Geometry check sheet. Reference: drawing and pictorial views, mm from the part's lowest x, y, z. A direction names the side the tool comes from. Give positions to 0.01 mm unless a question says otherwise; leave off trailing zeros. Write each loop counter-clockwise with the first axis right and the second up, starting at its lowest first coordinate (ties: lowest second). Pieces come first, ordered by that corner, then holes. Notation, with made-up numbers: M -13.5,-7.5 L 37.5,-7.5 A21 ccw 37.5,5.5 Z; hole C 88,55 d10. An arc over 180 degrees is marked long. One line per item, written item: value. Start each with the question number.
1. Cross-section at A-A on x = 14. Record the cut outline in (y, z).
2. Cross-section at B-B on z = 20.5. Record the cut outline in (x, y), then the cut area to 3 significant figures.
3. Scan lines: line 1 (X direction, y = 20.4, z = 10); line 2 (Y direction, x = 4.75, z = 17); line 3 (Z direction, x = 15, y = 26). Record each from-to range of solid material in increasing order.
4. Gauge pin test, flat ends, axial feed: pin 1 (11.5 mm diameter, centred on x = 14, z = 10, fed in from -Y); pin 2 (4.5 mm diameter, centred on y = 22, z = 16, fed in from +X); pin 3 (3 mm diameter, centred on x = 20, y = 17, fed in from -Z); pin 4 (3 mm diameter, centred on x = 13.5, z = 8.5, fed in from -Y). Record the tip position at first contact, or that the pin passes through.
5. Tool access check on the marked faces 4, 5 and 6. Record the directions out of +Z, -Z, +X, -X, +Y, -Y that give a thin tool (end or side, any length) a straight path to the whole face; none if there is none.
6. Cross-section at D-D on y = 21. Record the cut outline in (x, z).
7. Cross-section at C-C on z = 11. Record the cut outline in (x, y).
8. Release check for a two-part mould opening along Y. For the marked faces 1, 2 and 3 record: pulls with the +Y half, pulls with the -Y half, needs draft (parallel to the pull), parting line crosses it, or undercut.
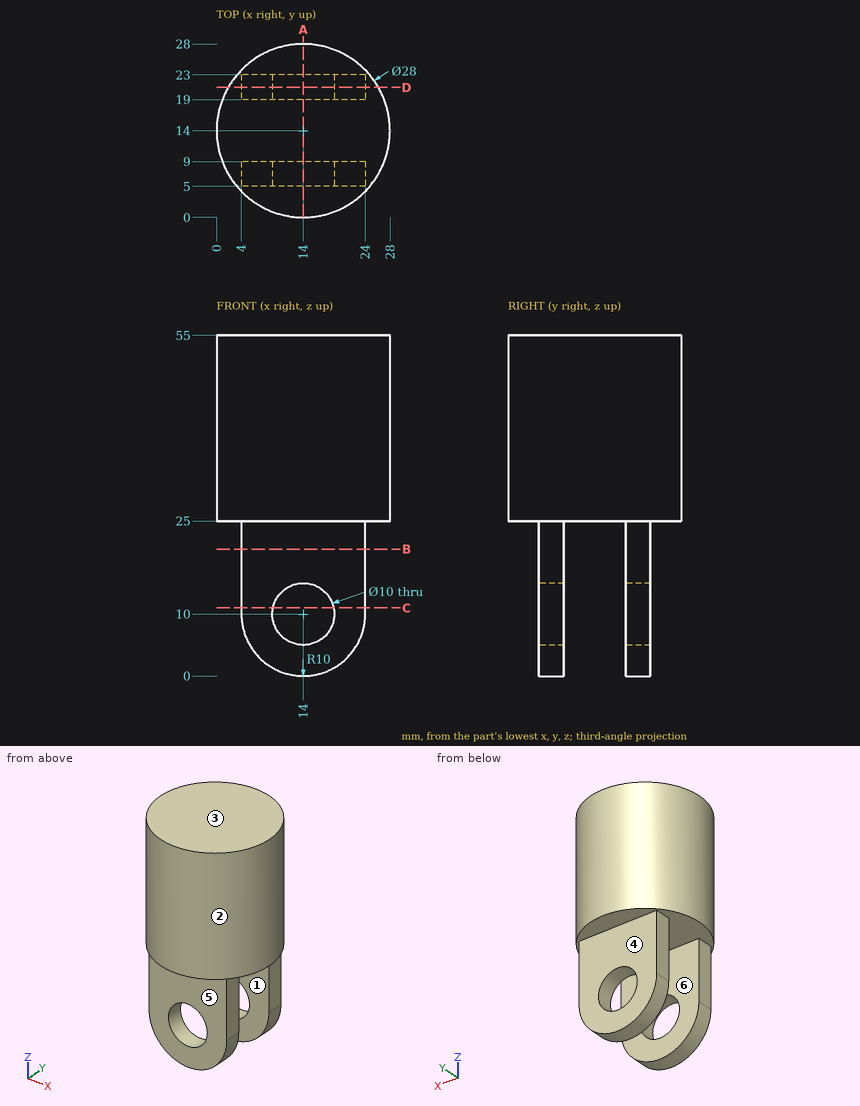
Report:
1. outline: M 0,25 L 5,25 L 5,15 L 9,15 L 9,25 L 19,25 L 19,15 L 23,15 L 23,25 L 28,25 L 28,55 L 0,55 Z; M 5,0 L 9,0 L 9,5 L 5,5 Z; M 19,0 L 23,0 L 23,5 L 19,5 Z
2. outline: M 4,5 L 24,5 L 24,9 L 4,9 Z; M 4,19 L 24,19 L 24,23 L 4,23 Z
2. area: 160 mm^2
3. line 1: x = 4 to 9, 19 to 24
3. line 2: y = 5 to 9, 19 to 23
3. line 3: z = 25 to 55
4. pin 1: stops at y = 5
4. pin 2: stops at x = 24
4. pin 3: stops at z = 25
4. pin 4: passes through
5. face 4: -Z, +X, -X, +Y
5. face 5: -Z, +X, -X, -Y
5. face 6: -Z, +X, -X
6. outline: M 1.88,25 L 4,25 L 4,10 A10 ccw 24,10 L 24,25 L 26.12,25 L 26.12,55 L 1.88,55 Z; hole C 14,10 d10
7. outline: M 4,5 L 9.1,5 L 9.1,9 L 4,9 Z; M 4,19 L 9.1,19 L 9.1,23 L 4,23 Z; M 18.9,5 L 24,5 L 24,9 L 18.9,9 Z; M 18.9,19 L 24,19 L 24,23 L 18.9,23 Z
8. face 1: undercut
8. face 2: parting line crosses it
8. face 3: needs draft
